Design review of the part built by this model. Coordinates are the model's own, in mm. Face numbers are marked on the shaded views. A direction names the side the tool comes from. Coordinates: 2 decimals unless noted, no trailing zeros. Write each loop counter-clockwise with the first axis right and the second up, starting at its lowest first coordinate (ties: lowest second). Pieces come first, ordered by that corner, then holes.
Q1. For pin 1 Ø3 at (y, z) = (-25, 12) entering from +X; pin 2 Ø21 at (y, z) = (33, 17.5) entering from -X; pin 3 Ø0.9 at (x, y) = (-32.5, -10) entering from +Z, all flat-tipped, find the tip position at first contact; note any pin that passes through.
Q2. For the marked faces 1, 2, 3, 4 and 5, list the 3-axis set-ups (+Z, -Z, +X, -X, +Y, -Y) from which the entire face can be reached by the end or side of a thin tool; tool diameter is ignored.
Q3. For L1, parallel to Y at x = -52, z = 42; L2, parallel to Y at x = 0, z = 4.25; L3, parallel to Y at x = -14.5, z = 41, list the stretches that pass through material, from the lowest coordinate up.
Q4. Take a section at C-C, the plane x = 0. Write out the cut boundary in (y, z).
Q5. The part is to be moulded in two halves that separate along Z. For the marked faces 6, 7 and 8, say which applies: released by +Z, released by -Z, zero draft, split by the parting line, or undercut.
Autodesk Fusion 360 part; units mm, degrees
sketch "Sketch3" plane through (0, 0, 0) normal (0, 0, 1) x (1, 0, 0)
  line L0 (33.5, -44) -> (-33.5, -44)
  line L1 (-33.5, -44) -> (-33.5, 44)
  line L2 (-33.5, 44) -> (33.5, 44)
  line L3 (33.5, -44) -> (-33.5, 44) construction
  line L4 (-33.5, -44) -> (33.5, 44) construction
  circle A0 centre (0, 25) radius 5
  circle A1 centre (0.3763, -25) radius 5
  line L5 (33.5, -44) -> (57.4793, -11.2043)
  line L6 (57.476, 11.2288) -> (33.5, 44)
  arc A2 (57.4793, -11.2043) -> (57.476, 11.2288) centre (42.1418, 0.01) ccw
  line L7 (33.5, 44) -> (33.5, -44)
  dimension "d5" = 67
  dimension "d6" = 88
  dimension "d7" = 10
  dimension "d8" = 10
  dimension "d9" = 50
  dimension "d10" = 19
  dimension "d55" = 19
extrude "Extrude1" add sketch "Sketch3" along normal blind 10 contours L0 L1 L2 L7 makes body 1
sketch "Sketch4" plane through (0, 0, 0) normal (0, 0, 1) x (1, 0, 0)
  line L0 (-33.5117, 43.8664) -> (-46.5117, 43.8664)
  line L1 (-46.5117, -44.1336) -> (-33.5117, -44.1336)
  line L2 (-33.5117, -44.1336) -> (-33.5117, 43.8664)
  line L3 (-46.5117, 43.8664) -> (-46.5117, 24.9992)
  line L4 (-46.5117, -24.9992) -> (-46.5117, -44.1336)
  arc A0 (-52.5605, 18.9994) -> (-52.5605, -18.9994) centre (-52.715, 0) ccw
  circle A1 centre (-52.715, 0) radius 9.5
  arc A2 (-52.5605, 18.9994) -> (-46.5117, 24.9992) centre (-52.5117, 24.9992) ccw
  arc A3 (-46.5117, -24.9992) -> (-52.5605, -18.9994) centre (-52.5117, -24.9992) ccw
  dimension "d16" = 19
  dimension "d17" = 19
  dimension "d18" = 6
  dimension "d19" = 6
extrude "Extrude2" add sketch "Sketch4" along normal blind 50 separate body makes body 2
sketch "Sketch5" plane through (-33.5117, 0, 0) normal (1, 0, 0) x (0, 1, 0)
  line L0 (-44.1336, 0) -> (43.8664, 0)
  line L1 (43.8664, 0) -> (43.8664, 50)
  line L2 (43.8664, 50) -> (-44.1336, 50)
  line L3 (-44.1336, 50) -> (-44.1336, 0)
  line L4 (-19.1336, 49.9963) -> (18.8664, 49.9963)
  line L5 (18.8664, 49.9963) -> (18.8664, 9.9944)
  line L6 (18.8664, 9.9944) -> (-19.1336, 9.9944)
  line L7 (-19.1336, 9.9944) -> (-19.1336, 49.9963)
  dimension "d22" = 38
  dimension "d23" = 25
extrude "Extrude4" add sketch "Sketch5" along normal blind 3 contours L4 L5 L6 L7 bodies 2
fillet "Fillet2" radius 3 1 edges at (-33.5117, -19.1336, 29.9954) on bodies 2
fillet "Fillet3" radius 3 1 edges at (-33.5117, 18.8664, 29.9954) on bodies 2
extrude "Extrude3" cut sketch "Sketch5" along normal blind 3 contours L4 L5 L6 L7 bodies 1
sketch "Sketch8" plane through (0, 0, 10) normal (0, 0, 1) x (-1, 0, 0)
  line L0 (30.5117, 19.1336) -> (33.5, 19.1336)
  line L1 (33.5, 19.1336) -> (33.5, 44)
  line L2 (33.5, 44) -> (-33.5, 44)
  line L3 (-33.5, -44) -> (33.5, -44)
  line L4 (33.5, -44) -> (33.5, -18.8664)
  line L5 (33.5, -18.8664) -> (30.5117, -18.8664)
  line L6 (30.5117, -18.8664) -> (30.5117, 19.1336)
  circle A0 centre (-0.3763, 25) radius 5
  circle A1 centre (0, -25) radius 5
  line L7 (30.5117, -4.8664) -> (-33.5, -4.8664)
  line L8 (-33.5, -4.8664) -> (-33.5, 5.1336)
  line L9 (-33.5, 5.1336) -> (30.5117, 5.1336)
  line L10 (30.5117, 5.1336) -> (30.5117, -4.8664)
  line L11 (-33.5, 44) -> (-33.5, -44)
  dimension "d38" = 14
  dimension "d39" = 10
extrude "Extrude5" add sketch "Sketch8" along normal blind 40 contours L6 L7 L8 L9 L10 L11 bodies 1 2
chamfer "Chamfer1" distance 60 angle 33.5 1 edges at (33.5, -0.1336, 50) measured on face at (12.1628, -1.8003, 50) on bodies 1
extrude "Extrude7" add sketch "Sketch3" along normal blind 10 contours L5 L6 A2 L7 bodies 1
fillet "Fillet8" radius 13 1 edges at (33.5, -44, 5) on bodies 1
fillet "Fillet9" radius 13 1 edges at (33.5, 44, 5) on bodies 1
equation "d10 = ( ( 88 - 50 ) / 2 ) * 1 mm"
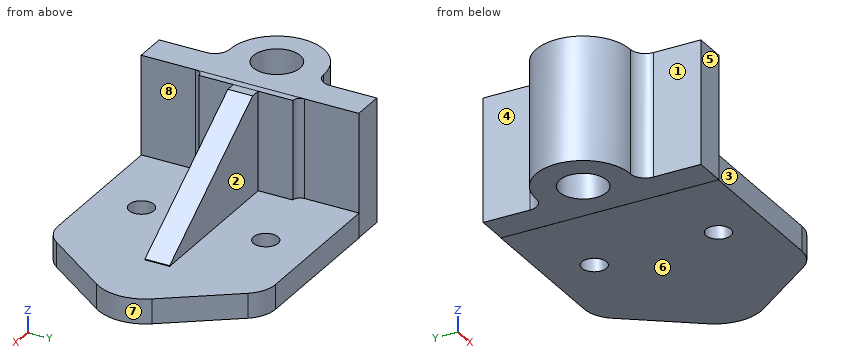
Responses:
1. pin 1: stops at x = -33.51
1. pin 2: stops at x = -47.06
1. pin 3: stops at z = 50
2. face 1: +Z, -Z, -X, -Y
2. face 2: +Z, +X, +Y
2. face 3: +Z, -Z, +X, -Y
2. face 4: +Z, -Z, -X, +Y
2. face 5: +Z, -Z, +X, -X, -Y
3. L1: y = -19.02 to -9.47, 9.47 to 19.02
3. L2: y = -44 to -29.99, -20.01 to 20, 30 to 44
3. L3: y = -5.13 to 4.87
4. outline: (-44, 0) - (-29.99, 0) - (-29.99, 10) - (-44, 10) - close; (-20.01, 0) - (20, 0) - (20, 10) - (4.87, 10) - (4.87, 32.46) - (-5.13, 32.46) - (-5.13, 10) - (-20.01, 10) - close; (30, 0) - (44, 0) - (44, 10) - (30, 10) - close
5. face 6: released by -Z
5. face 7: zero draft
5. face 8: undercut
